Build history of the part. All positions in model axes, mm. Face numbers are marked on the shaded views. A direction names the side the tool comes from. Give positions to 0.01 mm unless a question says otherwise; leave off trailing zeros. Loops run counter-clockwise (first coordinate to the right, second up) from the corner with the lowest first, then second, coordinate; pieces in that order, holes last.
1) Band-saw the part on D-D on z = 16.5. List the corners of the cut face in (x, y), then the cut area to 3 significant figures.
2) Wall check: line 1 (X direction, y = 1, z = 12.7) (3 decimals); line 2 (Y direction, x = 0.8, z = 12.7). Give the ranges that are in metal, low to high.
3) Band-saw the part on A-A on z = 12.7. List the corners of the cut face in (x, y) (1 decimal).
4) Flat gauge pins, fed straight in: P1, Ø3, axis at y = 8.5, z = 17.5, coming from the +X side; P2, Ø1, axis at x = 17, z = 3, coming from the +Y side. Where does each tip first touch, or does it go through?
5) Band-saw the part on B-B on x = 12.7. List the corners of the cut face in (y, z) (1 decimal).
6) 3-axis set-ups, long thin cutter, end or side, ignore diameter. For the marked faces 1 and 2: which of +Z, -Z, +X, -X, +Y, -Y reach the whole face in a straight line?
7) Band-saw the part on C-C on y = 15.75. List the corners of the cut face in (x, z), then the cut area to 3 significant figures.
```python
from build123d import *

# Parameters (mm, degrees)
BOSS_EXTRUDE1_DEPTH = 25.4
SKETCH2_R           = 3.175
CUT_EXTRUDE1_DEPTH  = 25.4
SKETCH3_R           = 6.35
CUT_EXTRUDE2_DEPTH  = 25.4


with BuildPart() as part:
    # Sketch1 → Boss-Extrude1 (new body)
    with BuildSketch(Plane.XY):
        Polygon((0, 0), (0, 25.4), (1.5875, 25.4), (1.5875, 1.5875), (25.4, 1.5875), (25.4, 0), align=None)
    extrude(amount=BOSS_EXTRUDE1_DEPTH)

    # Sketch2 → Cut-Extrude1 (cut)
    with BuildSketch(Plane(origin=(0, 1.5875, 0), x_dir=(1, 0, 0), z_dir=(0, 1, 0))):
        with Locations((12.7, -12.7)):
            Circle(SKETCH2_R)
    extrude(amount=-CUT_EXTRUDE1_DEPTH, mode=Mode.SUBTRACT)

    # Sketch3 → Cut-Extrude2 (cut)
    with BuildSketch(Plane(origin=(1.5875, 0, 0), x_dir=(0, 0, -1), z_dir=(1, 0, 0))):
        with Locations((-12.7, 13.49375)):
            Circle(SKETCH3_R)
    extrude(amount=-CUT_EXTRUDE2_DEPTH, mode=Mode.SUBTRACT)


solid = part.part
```
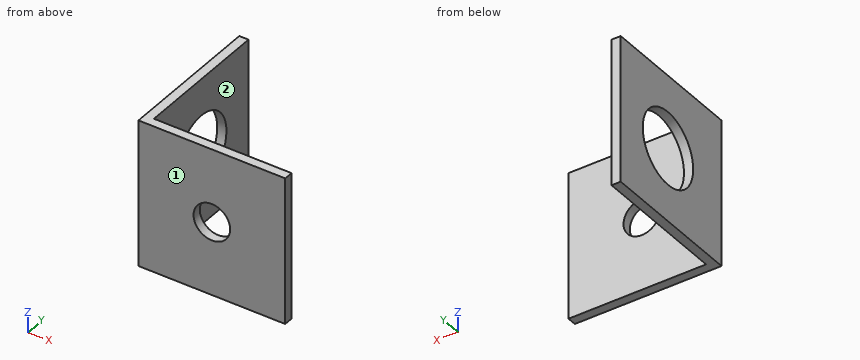
Findings below:
1. outline: (0, 0) - (25.4, 0) - (25.4, 1.59) - (1.59, 1.59) - (1.59, 8.41) - (0, 8.41) - close; (0, 18.58) - (1.59, 18.58) - (1.59, 25.4) - (0, 25.4) - close
1. area: 62.0 mm2
2. line 1: x = 0 to 9.525, 15.875 to 25.4
2. line 2: y = 0 to 7.14, 19.84 to 25.4
3. outline: (0, 0) - (9.5, 0) - (9.5, 1.6) - (1.6, 1.6) - (1.6, 7.1) - (0, 7.1) - close; (0, 19.8) - (1.6, 19.8) - (1.6, 25.4) - (0, 25.4) - close; (15.9, 0) - (25.4, 0) - (25.4, 1.6) - (15.9, 1.6) - close
4. P1: stops at x = 1.59
4. P2: stops at y = 1.59
5. outline: (0, 0) - (1.6, 0) - (1.6, 9.5) - (0, 9.5) - close; (0, 15.9) - (1.6, 15.9) - (1.6, 25.4) - (0, 25.4) - close
6. face 1: +Z, -Z, +X, -X, -Y
6. face 2: +Z, -Z, +X, +Y
7. outline: (0, 0) - (1.59, 0) - (1.59, 6.76) - (0, 6.76) - close; (0, 18.64) - (1.59, 18.64) - (1.59, 25.4) - (0, 25.4) - close
7. area: 21.5 mm2
